For this review, use the dimensioned drawing (mm, ordinates from the lowest corner) and the shaded views. A direction names the side the tool comes from. Round coordinates to 2 decimals unless told otherwise and drop trailing zeros. Write each loop counter-clockwise with the first axis right and the second up, starting at its lowest first coordinate (ties: lowest second). Pieces come first, ordered by that corner, then holes. Notation, with made-up numbers: M 88.25,0.5 L 125.25,0.5 A23 cw 125.25,30.5 Z; hole C -1.75,-7.75 d6. An arc over 180 degrees is marked long. Use CSV: the item, a comma, the result in double quotes.
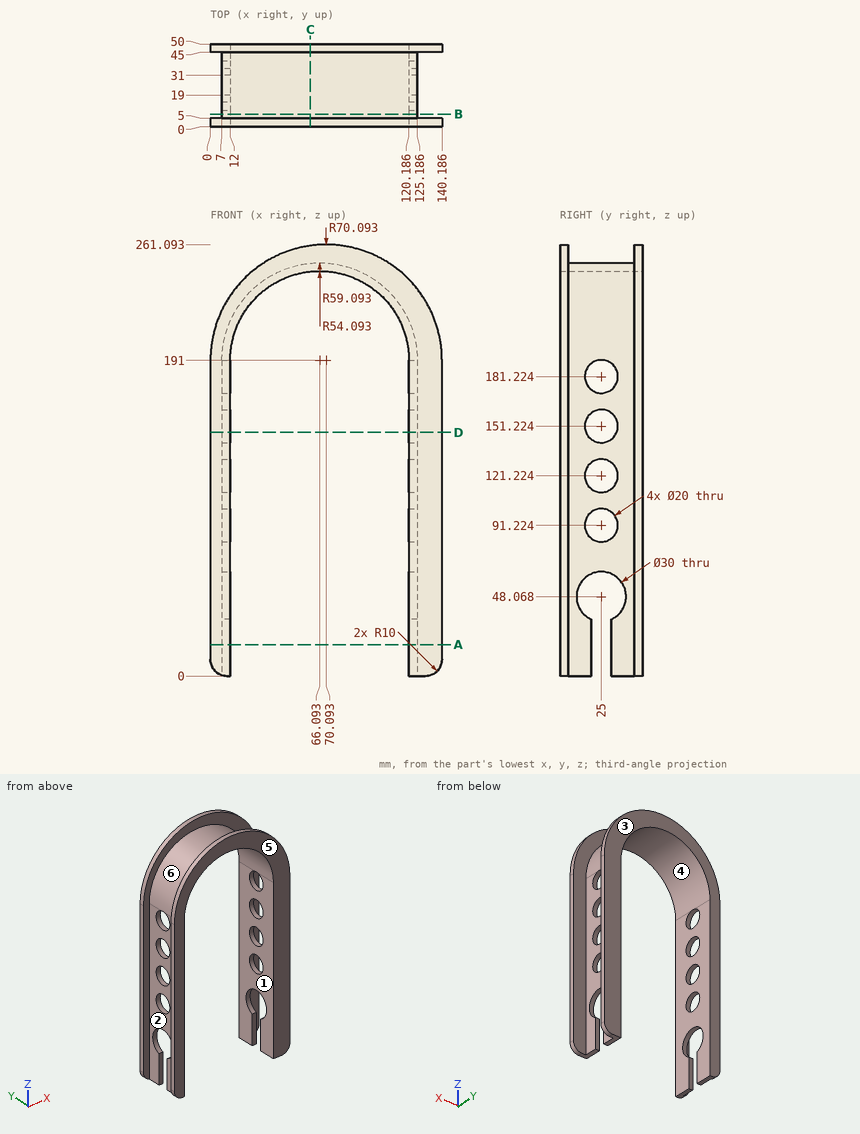
1) Add section A-A on z = 19. Write out the cut boundary in (x, y), then the cut area to 3 significant figures.
Answers:
outline,"M 0,0 L 12,0 L 12,19 L 7,19 L 7,5 L 0,5 Z; M 0,45 L 7,45 L 7,31 L 12,31 L 12,50 L 0,50 Z; M 120.19,0 L 140.19,0 L 140.19,5 L 125.19,5 L 125.19,19 L 120.19,19 Z; M 120.19,31 L 125.19,31 L 125.19,45 L 140.19,45 L 140.19,50 L 120.19,50 Z"
area,"600 mm²"
2) Machinability: for the marked faces 1, 2 and 3, which of the approach directions +Z, -Z, +X, -X, +Y, -Y give a long, thin tool a straight path to every point of the face, cutting with its end or side? Answer none if there is none.
Answers:
face 1,"-Z, +Y, -Y"
face 2,"+Z, -Z, -X"
face 3,"+Z, -Z, +X, -X, +Y"
3) Add section D-D on z = 147.5. Write out the cut boundary in (x, y).
Answers:
outline,"M 0,0 L 12,0 L 12,15.72 L 7,15.72 L 7,5 L 0,5 Z; M 0,45 L 7,45 L 7,34.28 L 12,34.28 L 12,50 L 0,50 Z; M 120.19,0 L 140.19,0 L 140.19,5 L 125.19,5 L 125.19,15.72 L 120.19,15.72 Z; M 120.19,34.28 L 125.19,34.28 L 125.19,45 L 140.19,45 L 140.19,50 L 120.19,50 Z"
4) The part is to be moulded in two halves that separate along X. For the marked faces 4, 5 and 6, say which applies: released by +X, released by -X, zero draft, split by the parting line, or undercut.
Answers:
face 4,"undercut"
face 5,"zero draft"
face 6,"split by the parting line"
5) Add section C-C on x = 60.5. Write out the cut boundary in (y, z).
Answers:
outline,"M 0,244.8 L 50,244.8 L 50,260.43 L 45,260.43 L 45,249.83 L 5,249.83 L 5,260.43 L 0,260.43 Z"
6) Wall thickness on line 1 along X through (y, z) = (9, 94.5); line 2 along Z through (x, y) = (67, 6) (1 decimal); line 3 along X through (y, z) = (28.5, 225) (1 decimal): over which ranges is each line inside the solid? List them lowest first. Write a range as [from, to].
Answers:
line 1,"[7, 12], [120.19, 125.19]"
line 2,"[245.1, 250.1]"
line 3,"[17.8, 24], [108.2, 114.4]"
7) For pin 1 Ø4 at (x, y) = (65, 7.5) entering from -Z (1 decimal); pin 2 Ø1 at (x, y) = (98, 17) entering from -Z; pin 3 Ø6 at (y, z) = (25.5, 101) entering from -X; pin 4 Ø18 at (y, z) = (25, 151.22) entering from +X, all flat-tipped, find the tip position at first contact; note any pin that passes through.
Answers:
pin 1,"z = 245"
pin 2,"z = 234.31"
pin 3,"x = 7"
pin 4,"through"
8) Add section B-B on y = 7.5. Write out the cut boundary in (x, z), then the cut area to 3 significant figures.
Answers:
outline,"M 7,0.46 A10 ccw 10,0 L 12,0 L 12,191 A54.09 cw 120.19,191 L 120.19,0 L 125.19,0 L 125.19,191 A59.09 ccw 7,191 Z"
area,"2,800 mm²"
